from build123d import *

# Parameters (mm, degrees)
SKETCH2_R           = 14
SKETCH2_R_2         = 11
BOSS_EXTRUDE1_DEPTH = 12
SKETCH3_R           = 17
SKETCH3_R_2         = 14
BOSS_EXTRUDE2_DEPTH = 8.5
SKETCH4_R           = 2.5
SKETCH4_R_2         = 17
BOSS_EXTRUDE3_DEPTH = 3.5
FILLET1_R           = 1.5
FILLET2_R           = 7


with BuildPart() as part:
    # Sketch2 → Boss-Extrude1 (new body)
    with BuildSketch(Plane(origin=(0, 0, 0), x_dir=(1, 0, 0), z_dir=(0, 1, 0))):
        with Locations(Location((0, 0, 0), (0, 0, 270))):
            Circle(SKETCH2_R)
        with Locations(Location((0, 0, 0), (0, 0, 270))):
            Circle(SKETCH2_R_2, mode=Mode.SUBTRACT)
    extrude(amount=BOSS_EXTRUDE1_DEPTH)

    # Sketch3 → Boss-Extrude2 (add)
    with BuildSketch(Plane(origin=(0, 0, 0), x_dir=(1, 0, 0), z_dir=(0, 1, 0))):
        with Locations(Location((0, 0, 0), (0, 0, 270))):
            Circle(SKETCH3_R)
        with Locations(Location((0, 0, 0), (0, 0, 270))):
            Circle(SKETCH3_R_2, mode=Mode.SUBTRACT)
    extrude(amount=BOSS_EXTRUDE2_DEPTH)

    # Sketch4 → Boss-Extrude3 (add)
    with BuildSketch(Plane(origin=(0, 0, 0), x_dir=(1, 0, 0), z_dir=(0, 1, 0))):
        with BuildLine():
            ThreePointArc((-18.361144712, 13.004551698), (-22.5, 0), (-18.361144712, -13.004551698))
            ThreePointArc((-18.361144712, -13.004551698), (-18.077090702, -22.033356344), (-9.166775866, -20.547997962))
            ThreePointArc((-9.166775866, -20.547997962), (0, -22.5), (9.166775866, -20.547997962))
            ThreePointArc((9.166775866, -20.547997962), (18.077090702, -22.033356344), (18.361144712, -13.004551698))
            ThreePointArc((18.361144712, -13.004551698), (22.5, 0), (18.361144712, 13.004551698))
            ThreePointArc((18.361144712, 13.004551698), (18.077090702, 22.033356344), (9.166775866, 20.547997962))
            ThreePointArc((9.166775866, 20.547997962), (0, 22.5), (-9.166775866, 20.547997962))
            ThreePointArc((-9.166775866, 20.547997962), (-18.077090702, 22.033356344), (-18.361144712, 13.004551698))
        make_face()
        with Locations(Location((-14.271387396, 17.394755008, 0), (0, 0, 270))):
            Circle(SKETCH4_R, mode=Mode.SUBTRACT)
        with Locations(Location((14.271387396, 17.394755008, 0), (0, 0, 270))):
            Circle(SKETCH4_R, mode=Mode.SUBTRACT)
        with Locations(Location((-14.271387396, -17.394755008, 0), (0, 0, 270))):
            Circle(SKETCH4_R, mode=Mode.SUBTRACT)
        with Locations(Location((14.271387396, -17.394755008, 0), (0, 0, 270))):
            Circle(SKETCH4_R, mode=Mode.SUBTRACT)
        with Locations(Location((0, 0, 0), (0, 0, 270))):
            Circle(SKETCH4_R_2, mode=Mode.SUBTRACT)
    extrude(amount=BOSS_EXTRUDE3_DEPTH)

    # Fillet1
    fillet1_edges = [part.edges().sort_by_distance(p)[0] for p in [
        (0, 3.5, -17),
    ]]
    fillet(fillet1_edges, radius=FILLET1_R)

    # Fillet2
    fillet2_edges = [part.edges().sort_by_distance(p)[0] for p in [
        (-9.166775866, 1.75, 20.547997962),
        (9.166775866, 1.75, 20.547997962),
        (18.361144712, 1.75, 13.004551698),
        (18.361144712, 1.75, -13.004551698),
        (9.166775866, 1.75, -20.547997962),
        (-9.166775866, 1.75, -20.547997962),
        (-18.361144712, 1.75, -13.004551698),
        (-18.361144712, 1.75, 13.004551698),
    ]]
    fillet(fillet2_edges, radius=FILLET2_R)


solid = part.part
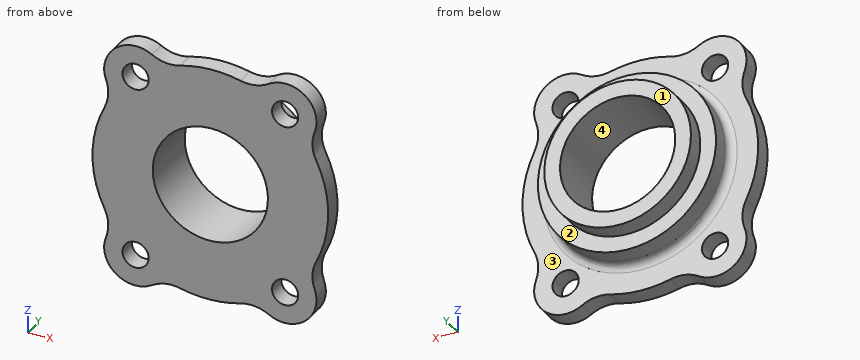
Check sheet for the modelled part. Datum: model origin and axes. Units: mm. Face numbers are marked on the shaded views. A direction names the side the tool comes from. Coordinates: 2 decimals unless noted, no trailing zeros. Write each loop counter-clockwise with the first axis right and the second up, starting at its lowest first coordinate (ties: lowest second). Pieces come first, ordered by that corner, then holes.
Item 1: Access from +Z, -Z, +X, -X, +Y, -Y to the whole of each face (thin tool, end or side, straight path). Record for the marked faces 1 and 2.
Numbers:
face 1: +Z, -Z, +X, -X, +Y
face 2: +Y
Item 2: Mould release check, pull along X, two halves, no side actions. Record for the marked faces 3 and 4: released by +X, released by -X, zero draft, split by the parting line, or undercut.
Numbers:
face 3: zero draft
face 4: undercut
Item 3: Cross-section at B-B on z = 0. Record the boundary of the cut face in (x, y).
Numbers:
outline: (-22.5, 0) - (-11, 0) - (-11, 12) - (-14, 12) - (-14, 8.5) - (-17, 8.5) - (-17, 5) arc R1.5 cw to (-18.5, 3.5) - (-22.5, 3.5) - close; (11, 0) - (22.5, 0) - (22.5, 3.5) - (18.5, 3.5) arc R1.5 cw to (17, 5) - (17, 8.5) - (14, 8.5) - (14, 12) - (11, 12) - close
Item 4: Depth check by flat-ended pin: pin 1 Ø1 at (y, z) = (10, -6) entering from +X; pin 2 Ø6.5 at (x, z) = (-14.27, -17.39) entering from -Y; pin 3 Ø4 at (y, z) = (7, -0.5) entering from -X; pin 4 Ø6.5 at (x, z) = (-14.27, 17.39) entering from +Y. Enter the tip coordinate at first touch or a pass-through.
Numbers:
pin 1: stops at x = 12.87
pin 2: stops at y = 0
pin 3: stops at x = -17
pin 4: stops at y = 3.5
Item 5: Scan lines: probe 1 along X at (y, z) = (2.75, -19); probe 2 along X at (y, z) = (8, 0); probe 3 along Z at (x, y) = (14, 0.75). Record each from-to range of solid material in increasing order.
Numbers:
probe 1: x = -20.05 to -16.19, -12.35 to 12.35, 16.19 to 20.05
probe 2: x = -17 to -11, 11 to 17
probe 3: z = -23.39 to -19.88, -14.91 to 14.91, 19.88 to 23.39
Item 6: Cross-section at C-C on y = 9.25. Record the boundary of the cut face in (x, z).
Numbers:
outline: circle Ø28 at (0, 0); hole circle Ø22 at (0, 0)
Item 7: Cross-section at D-D on y = 1. Count the separate pieces of the cut face and the enclosed holes in it, then the cut area to 3 significant figures.
Numbers:
separate pieces: 1
enclosed holes: 5
area: 1,390 mm2
Item 8: Cross-section at A-A on x = 0. Record the boundary of the cut face in (y, z).
Numbers:
outline: (0, -22.5) - (3.5, -22.5) - (3.5, -18.5) arc R1.5 cw to (5, -17) - (8.5, -17) - (8.5, -14) - (12, -14) - (12, -11) - (0, -11) - close; (0, 11) - (12, 11) - (12, 14) - (8.5, 14) - (8.5, 17) - (5, 17) arc R1.5 cw to (3.5, 18.5) - (3.5, 22.5) - (0, 22.5) - close
